Autodesk Inventor part; units mm, degrees
ref_plane "YZ Plane" through (0, 0, 0) normal (1, 0, 0) x (0, 1, 0)
ref_plane "XZ Plane" through (0, 0, 0) normal (0, 1, 0) x (-1, 0, 0)
ref_plane "XY Plane" through (0, 0, 0) normal (0, 0, 1) x (1, 0, 0)
sketch "Sketch1" plane through (0, 0, 0) normal (1, 0, 0) x (0, 1, 0)
  line L0 (0, 0) -> (25.4, 0)
  line L1 (25.4, 0) -> (25.4, -25.4)
  line L2 (25.4, -25.4) -> (23.8252, -25.4)
  line L3 (0, -1.5748) -> (0, 0)
  line L4 (25.4, 0) -> (22.225, 0) construction
  line L5 (22.225, 0) -> (22.225, -3.175) construction
  line L6 (22.225, -3.175) -> (25.4, -3.175) construction
  line L7 (25.4, -3.175) -> (25.4, 0) construction
  line L8 (25.4, -25.4) -> (22.225, -25.4) construction
  line L9 (0, 0) -> (0, -3.175) construction
  line L10 (1.6002, -3.175) -> (20.6248, -3.175)
  line L11 (22.225, -23.7998) -> (22.225, -4.7752)
  arc A0 (22.225, -23.7998) -> (23.8252, -25.4) centre (23.8252, -23.7998) ccw
  arc A1 (0, -1.5748) -> (1.6002, -3.175) centre (1.6002, -1.5748) ccw
  arc A2 (22.225, -4.7752) -> (20.6248, -3.175) centre (20.6248, -4.7752) ccw
  point P0 (0, -25.4)
  dimension "d0" = 25.4
  dimension "d1" = 25.4
  dimension "d2" = 3.175
  dimension "d3" = 3.175
  dimension "d4" = 3.175
  dimension "d5" = 3.175
  dimension "d6" = 1.6002
  dimension "d7" = 1.6002
extrude "Extrusion1" add sketch "Sketch1" along normal blind 660.4
sketch "Sketch2" plane through (0, 25.4, 0) normal (0, 1, 0) x (1, 0, 0)
  line L0 (0, 25.4) -> (0, 23.7998)
  line L1 (0, 3.175) -> (660.4, 3.175)
  line L2 (0, 25.4) -> (25.4, 25.4)
  line L3 (25.4, 25.4) -> (25.4, 3.175)
  line L4 (25.4, 3.175) -> (0, 3.175)
  line L5 (0, 3.175) -> (0, 25.4)
  line L6 (660.4, 25.4) -> (635, 25.4)
  line L7 (635, 25.4) -> (635, 3.175)
  line L8 (635, 3.175) -> (660.4, 3.175)
  line L9 (660.4, 3.175) -> (660.4, 25.4)
  point P0 (0, 0)
  dimension "d10" = 25.4
  dimension "d11" = 25.4
  dimension "d12" = 22.225
extrude "Extrusion2" cut sketch "Sketch2" against normal blind 25.4
properties part number "24in1.0Lch" material "Steel, Mild"
Can you work these out from the model? Positions are in its coordinate system, mm. A direction names the side the tool comes from. Coordinates: 2 decimals unless noted, no trailing zeros. Loops run counter-clockwise (first coordinate to the right, second up) from the corner with the lowest first, then second, coordinate; pieces in that order, holes last.
Item 1: Suppose I cut it at A-A (x = 123). Please give me the cut outline in (y, z) (3 decimals), then the cut area to 3 significant figures.
Answers below:
outline: (0, -1.575) arc R1.6 ccw to (1.6, -3.175) - (20.625, -3.175) arc R1.6 cw to (22.225, -4.775) - (22.225, -23.8) arc R1.6 ccw to (23.825, -25.4) - (25.4, -25.4) - (25.4, 0) - (0, 0) - close
area: 151 mm2
Item 2: Please list where these lines run through material, in increasing order: L1, parallel to Y at x = 477, z = -20.5 (3 decimals); L2, parallel to Z at x = 554, y = 18 (3 decimals); L3, parallel to Y at x = 364, z = -2.
Answers below:
L1: y = 22.225 to 25.4
L2: z = -3.175 to 0
L3: y = 0.06 to 25.4
Item 3: I'm going to push flat-ended pins straight in: pin 1 (1 mm diameter, centred on x = 401.5, z = -11, fed in from -Y) (3 decimals); pin 2 (7 mm diameter, centred on x = 363, y = 12.5, fed in from -Z) (3 decimals); pin 3 (5.5 mm diameter, centred on y = 22, z = -11.5, fed in from +X). Where does each tip first touch, or does it pass through?
Answers below:
pin 1: stops at y = 22.225
pin 2: stops at z = -3.175
pin 3: stops at x = 635
Item 4: Which directions (+Z, -Z, +X, -X, +Y, -Y) give clear straight access to the entire face, cutting with the end or side of a thin tool? Please do faces 1 (the face through (326, 22.225, -14)), 2 (the face through (326, 25.4, -13)).
Answers below:
face 1: -Z, +X, -X, -Y
face 2: +Z, -Z, +X, -X, +Y
Item 5: Suppose I cut it at C-C (y = 15.5). Please give me the cut outline in (x, z) (3 decimals).
Answers below:
outline: (0, -3.175) - (660.4, -3.175) - (660.4, 0) - (0, 0) - close
Item 6: Suppose I cut it at B-B (z = -13.5). Please give me the cut outline in (x, y) (3 decimals).
Answers below:
outline: (25.4, 22.225) - (635, 22.225) - (635, 25.4) - (25.4, 25.4) - close
